Can you work these out from the model? Positions are in its coordinate system, mm. A direction names the side the tool comes from. Coordinates: 2 decimals unless noted, no trailing zeros. Order: outer loops, then holes, each group sorted by start corner. A loop starts at its lowest first (then second) coordinate and runs counter-clockwise, first axis right, second up. Notation, with made-up numbers: (35.5, -10) - (50.5, -10) arc R23 ccw to (50.5, 24) - close; hole circle Ø6 at (18.25, 6.25). An arc over 180 degrees is marked (long way). Use a Markdown table: item, result. Add a question column.
(1) If I drill on L1, parallel to Z at x = -148, y = 25; L2, parallel to Z at x = 105, y = 9; L3, parallel to X at y = 6, z = -192, over which ranges is the centre line in solid material (lowest first)? Write a range as [from, to].
(2) I want a section at D-D (z = 53). List the corners of the cut face in (x, y) for me.
(3) I want a section at A-A (z = 125). List the corners of the cut face in (x, y) for me, and give its area (3 significant figures).
(4) For pin 1 Ø3 at (y, z) = (34.9, -134.9) entering from -X, with a flat end and sliding along its axis, tell me the tip position at first contact or that it passes through.
(5) I want a section at B-B (x = -23). List the corners of the cut face in (y, z) for me, and give its area (3 significant figures).
(6) I want a section at C-C (y = 93). List the corners of the cut face in (x, z) for me.
(7) We'd pull the mould along Z, two halves only. Please class faces 1 (the flat face through (147, 40, 3)), 2 (the flat face through (-2, 83, -225)), 3 (the flat face through (150, 38, -3)): pulls with the +Z half, pulls with the -Z half, needs draft (parallel to the pull), parting line crosses it, or undercut.
(8) On a 3-axis mill with a long thin cutter (end or side, diameter ignored), from which of +Z, -Z, +X, -X, +Y, -Y can I reach the whole of each face in a straight line? I mean faces 4 (the flat face through (-150, 38, 3)), 5 (the flat face through (2, 83, -222)), 6 (the cylindrical face through (-148.479, 65.385, 97.496)). Say none if no direction works.
Autodesk Inventor part; units mm, degrees
ref_plane "YZ Plane" through (0, 0, 0) normal (1, 0, 0) x (0, 1, 0)
ref_plane "XZ Plane" through (0, 0, 0) normal (0, 1, 0) x (-1, 0, 0)
ref_plane "XY Plane" through (0, 0, 0) normal (0, 0, 1) x (1, 0, 0)
sketch "Sketch1" plane through (0, 0, 0) normal (0, 1, 0) x (-1, 0, 0)
  line L0 (-150, 225) -> (150, 225)
  line L1 (150, 225) -> (150, -225)
  line L2 (150, -225) -> (-150, -225)
  line L3 (-150, -225) -> (-150, 225)
  line L4 (-150, 225) -> (150, -225) construction
  line L5 (150, 225) -> (-150, -225) construction
  line L6 (147, -222) -> (147, 222)
  line L7 (147, 222) -> (-147, 222)
  line L8 (-147, 222) -> (-147, -222)
  line L9 (-147, -222) -> (147, -222)
  point P0 (0, 0)
  dimension "d0" = 300
  dimension "d1" = 450
  dimension "d4" = 3
extrude "Extrusion1" add sketch "Sketch1" along normal blind 3 contours L0 L1 L2 L3 | L9 L8 L7 L6
extrude "Extrusion2" add sketch "Sketch1" along normal blind 100
sketch "Sketch2" plane through (150, 0, 225) normal (1, 0, 0) x (0, 0, -1)
  line L0 (0, 0) -> (450, 0)
  line L1 (450, 0) -> (450, 100)
  line L2 (0, 100) -> (450, 100)
  line L3 (0, 0) -> (0, 100)
  line L4 (0, 25) -> (450, 25)
  circle A0 centre (100, 25) radius 14
  circle A1 centre (350, 25) radius 14
  line L5 (100, 25) -> (109.8995, 34.8995) construction
  line L6 (100, 25) -> (114, 25) construction
  line L7 (225, 100) -> (225, 0) construction
  circle A2 centre (100, 25) radius 6
  circle A3 centre (350, 25) radius 6
  point P0 (90.1005, 34.8995)
  point P1 (90.1005, 15.1005)
  point P2 (109.8995, 15.1005)
  point P3 (340.1005, 34.8995)
  point P4 (359.8995, 34.8995)
  point P5 (359.8995, 15.1005)
  point P6 (340.1005, 15.1005)
  dimension "d7" = 28
  dimension "d8" = 28
  dimension "d9" = 45
  dimension "d12" = 360
  dimension "d14" = 12
  dimension "d15" = 12
hole "Hole1" at (150, 25, 125) at (150, 25, -125) direction (-1, 0, 0) diameter 12 end through all
hole "Hole2" at (150, 34.8995, 134.8995) at (150, 15.1005, 115.1005) at (150, 15.1005, 134.8995) at (150, 34.8995, 115.1005) at (150, 34.8995, -115.1005) at (150, 15.1005, -115.1005) at (150, 15.1005, -134.8995) at (150, 34.8995, -134.8995) direction (-1, 0, 0) diameter 3.5 end through all
sketch "Sketch3" plane through (0, 3, 0) normal (0, 1, 0) x (1, 0, 0)
  line L0 (-147, 222) -> (-147, -222)
  line L1 (-147, -222) -> (147, -222)
  line L2 (147, -222) -> (147, 222)
  line L3 (147, 222) -> (-147, 222)
  point P0 (0, 0)
sketch "Sketch4" plane through (0, 3, 0) normal (0, 1, 0) x (1, 0, 0)
  line L0 (-147, 222) -> (-147, -222)
  line L1 (147, -222) -> (147, 222)
  line L2 (150, 225) -> (-150, 225)
  line L3 (0, 225) -> (0, -313.1103)
  line L4 (-147, 0) -> (147, 0)
  point P0 (0, 0)
  point P1 (-202.9851, -76.8809)
  point P2 (132, 256.112)
  point P3 (-124.075, 248.076)
  point P4 (-124.075, -228.643)
  point P5 (147.6668, -220.1737)
  point P6 (132, 210)
  point P7 (-132, 210)
  point P8 (132, -210)
  point P9 (-132, -210)
  dimension "d30" = 132
  dimension "d31" = 210
hole "Hole3" at (132, 3, -210) at (-132, 3, -210) at (-132, 3, 210) at (132, 3, 210) direction (0, -1, 0) diameter 5 end through all
sketch "Sketch5" plane through (150, 0, 225) normal (1, 0, 0) x (0, 0, -1)
  circle A0 centre (359.8995, 34.8995) radius 1.75
  circle A1 centre (359.8995, 15.1005) radius 1.75
  circle A2 centre (340.1005, 15.1005) radius 1.75
  circle A3 centre (340.1005, 34.8995) radius 1.75
  circle A4 centre (109.8995, 34.8995) radius 1.75
  circle A5 centre (90.1005, 15.1005) radius 1.75
  circle A6 centre (109.8995, 15.1005) radius 1.75
  circle A7 centre (90.1005, 34.8995) radius 1.75
  circle A8 centre (350, 25) radius 6
  circle A9 centre (100, 25) radius 6
  line L0 (0, 0) -> (450, 0)
  line L1 (450, 0) -> (450, 100)
  line L2 (0, 100) -> (450, 100)
  line L3 (0, 0) -> (0, 100)
  point P0 (225, 0)
  point P1 (225, 65)
  point P2 (225, 65)
sketch "Sketch6" plane through (150, 0, 225) normal (1, 0, 0) x (0, 0, -1)
  circle A0 centre (359.8995, 34.8995) radius 1.75
  circle A1 centre (359.8995, 15.1005) radius 1.75
  circle A2 centre (340.1005, 15.1005) radius 1.75
  circle A3 centre (340.1005, 34.8995) radius 1.75
  circle A4 centre (109.8995, 34.8995) radius 1.75
  circle A5 centre (90.1005, 15.1005) radius 1.75
  circle A6 centre (109.8995, 15.1005) radius 1.75
  circle A7 centre (90.1005, 34.8995) radius 1.75
  circle A8 centre (350, 25) radius 6
  circle A9 centre (100, 25) radius 6
  line L0 (0, 0) -> (450, 0)
  line L1 (450, 0) -> (450, 100)
  line L2 (0, 100) -> (450, 100)
  line L3 (0, 0) -> (0, 100)
  point P0 (225, 0)
sketch "Sketch7" plane through (150, 0, 225) normal (1, 0, 0) x (0, 0, -1)
  line L0 (145, 65.0001) -> (305, 65.0001) construction
  line L1 (145, 47.5001) -> (305, 47.5001)
  line L2 (305, 82.5001) -> (145, 82.5001)
  arc A0 (145, 82.5001) -> (145, 47.5001) centre (145, 65.0001) ccw
  arc A1 (305, 47.5001) -> (305, 82.5001) centre (305, 65.0001) ccw
  point P0 (225, 0)
  point P1 (225, 65.0001)
  dimension "d42" = 80
  dimension "d43" = 35
extrude "Extrusion3" cut sketch "Sketch7" against normal through all
sketch "Sketch8" plane through (150, 0, 225) normal (1, 0, 0) x (0, 0, -1)
  line L0 (145, 82.5001) -> (305, 82.5001)
  arc A0 (305, 47.5001) -> (305, 82.5001) centre (305, 65.0001) ccw
  line L1 (305, 47.5001) -> (145, 47.5001)
  arc A1 (145, 82.5001) -> (145, 47.5001) centre (145, 65.0001) ccw
  circle A2 centre (359.8995, 34.8995) radius 1.75
  circle A3 centre (359.8995, 15.1005) radius 1.75
  circle A4 centre (340.1005, 15.1005) radius 1.75
  circle A5 centre (340.1005, 34.8995) radius 1.75
  circle A6 centre (109.8995, 34.8995) radius 1.75
  circle A7 centre (90.1005, 15.1005) radius 1.75
  circle A8 centre (109.8995, 15.1005) radius 1.75
  circle A9 centre (90.1005, 34.8995) radius 1.75
  circle A10 centre (350, 25) radius 6
  circle A11 centre (100, 25) radius 6
  line L2 (0, 0) -> (450, 0)
  line L3 (450, 0) -> (450, 100)
  line L4 (0, 100) -> (450, 100)
  line L5 (0, 0) -> (0, 100)
  point P0 (225, 0)
sketch "Sketch9" plane through (150, 0, -225) normal (0, 0, -1) x (-1, 0, 0)
  line L0 (0, 0) -> (300, 0)
  line L1 (300, 0) -> (300, 100)
  line L2 (0, 100) -> (300, 100)
  line L3 (0, 0) -> (0, 100)
  line L4 (100, 75) -> (200, 75)
  line L5 (200, 75) -> (200, 25)
  line L6 (200, 25) -> (100, 25)
  line L7 (100, 25) -> (100, 75)
  line L8 (100, 75) -> (200, 25) construction
  line L9 (200, 75) -> (100, 25) construction
  point P0 (150, 0)
  point P1 (150, 50)
  point P2 (150, 50)
  dimension "d46" = 100
  dimension "d47" = 50
sketch "Sketch10" plane through (150, 0, -225) normal (0, 0, -1) x (-1, 0, 0)
  line L0 (100.0001, 70) -> (100.0001, 30)
  line L1 (105.0001, 25) -> (195.0038, 25)
  line L2 (200.0038, 30) -> (200.0038, 70)
  line L3 (195.0038, 75) -> (105.0001, 75)
  arc A0 (105.0001, 75) -> (100.0001, 70) centre (105.0001, 70) ccw
  arc A1 (100.0001, 30) -> (105.0001, 25) centre (105.0001, 30) ccw
  arc A2 (195.0038, 25) -> (200.0038, 30) centre (195.0038, 30) ccw
  arc A3 (200.0038, 70) -> (195.0038, 75) centre (195.0038, 70) ccw
  point P0 (150, 0)
  point P1 (200.0038, 75)
  point P2 (100.0038, 75)
  dimension "d48" = 100
  dimension "d49" = 5
extrude "Extrusion4" cut sketch "Sketch10" against normal blind 3
properties part number "AMR_Base_Box_V2"
Answers follow:
| question | item | result |
|---|---|---|
| 1 | L1 | z = [-225, -131], [-119, 119], [131, 225] |
| 1 | L2 | z = [-225, -222], [222, 225] |
| 1 | L3 | x = [-150, -147], [147, 150] |
| 2 | outline | (-150, 0) - (150, 0) - (150, 47.5) - (147, 47.5) - (147, 3) - (-147, 3) - (-147, 47.5) - (-150, 47.5) - close; (-150, 82.5) - (-147, 82.5) - (-147, 100) - (-150, 100) - close; (147, 82.5) - (150, 82.5) - (150, 100) - (147, 100) - close |
| 3 | outline | (-150, 0) - (150, 0) - (150, 19) - (147, 19) - (147, 3) - (-147, 3) - (-147, 19) - (-150, 19) - close; (-150, 31) - (-147, 31) - (-147, 100) - (-150, 100) - close; (147, 31) - (150, 31) - (150, 100) - (147, 100) - close |
| 3 | area | 1,410 mm² |
| 4 | pin 1 | passes through |
| 5 | outline | (0, -225) - (25, -225) - (25, -222) - (3, -222) - (3, 222) - (100, 222) - (100, 225) - (0, 225) - close; (75, -225) - (100, -225) - (100, -222) - (75, -222) - close |
| 5 | area | 1,780 mm² |
| 6 | outline | (-150, -225) - (150, -225) - (150, 225) - (-150, 225) - close; hole (-147, -222) - (147, -222) - (147, 222) - (-147, 222) - close |
| 7 | face 1 | undercut |
| 7 | face 2 | pulls with the -Z half |
| 7 | face 3 | needs draft |
| 8 | face 4 | +Z, -Z, -X, +Y, -Y |
| 8 | face 5 | +Y |
| 8 | face 6 | +X, -X |
